Build history of the part. All positions in model axes, mm. A direction names the side the tool comes from. Round coordinates to 2 decimals unless told otherwise and drop trailing zeros. Write each loop counter-clockwise with the first axis right and the second up, starting at its lowest first coordinate (ties: lowest second). Pieces come first, ordered by that corner, then holes. Notation, with made-up numbers: (-9, 1.5) -> (38, 1.5) arc R12 ccw to (38, 23.5) -> close; hole circle Ø2 at (11.5, 88). An arc over 180 degrees is marked (long way). Answer in a Markdown table with one row per item.
```python
from build123d import *

# Parameters (mm, degrees)
F0_R     = 7.5
F1_DEPTH = 4
F2_R     = 5
F3_DEPTH = 100
F4_W     = 4
F4_H     = 4
F5_DEPTH = 20
F6_W     = 10.298821
F6_H     = 32.871584
F7_DEPTH = 25


with BuildPart() as f1:
    # F0 (on Top) → F1 (new body)
    with BuildSketch(Plane.XY):
        Circle(F0_R)
    extrude(amount=F1_DEPTH)

    # F2 (on Top) → F3 (join)
    with BuildSketch(Plane.XY):
        Circle(F2_R)
    extrude(amount=F3_DEPTH)

    # F4 (on face) → F5 (join)
    with BuildSketch(Plane.XY.offset(100)):
        Rectangle(F4_W, F4_H)
    extrude(amount=F5_DEPTH)

    # F6 (on Top) → F7 (cut)
    with BuildSketch(Plane.XY):
        with Locations((12.149411, 0.144365)):
            Rectangle(F6_W, F6_H)
    extrude(amount=F7_DEPTH, mode=Mode.SUBTRACT)


solid = f1.part
```
Q1. Saw through at D-D on x = -6. Write the cut outline in (y, z), plus the area to 3 significant figures.
A:
| item | result |
|---|---|
| outline | (-4.5, 0) -> (4.5, 0) -> (4.5, 4) -> (-4.5, 4) -> close |
| area | 36.0 mm² |
Q2. Which spindle directions (+Z, -Z, +X, -X, +Y, -Y) get a long thin tool onto all of the face, cutting with end or side? Do faces 1 (the flat face through (-5.2, 0.1, 4)), 2 (the flat face through (2, 0, 110)), 3 (the flat face through (-2, 0, 110)). Say none if no direction does.
A:
| item | result |
|---|---|
| face 1 | +Z |
| face 2 | +Z, +X, +Y, -Y |
| face 3 | +Z, -X, +Y, -Y |
Q3. Wall check: line 1 (Z direction, x = 1.75, y = -5); line 2 (Z direction, x = 3, y = -0.25); line 3 (Y direction, x = -4.5, z = 21.5). Give the ranges that are in metal, low to high. Write a range as [from, to].
A:
| item | result |
|---|---|
| line 1 | [0, 4] |
| line 2 | [0, 100] |
| line 3 | [-2.18, 2.18] |
Q4. Drop flat-ended pins along their axis: P1, Ø3, axis at y = -0.5, z = 110, coming from the +X side; P2, Ø6, axis at x = 3.5, z = 55.5, coming from the -Y side; P3, Ø2, axis at x = -0.5, z = 110.5, coming from the +Y side. Give the stop position or say it passes through.
A:
| item | result |
|---|---|
| P1 | x = 2 |
| P2 | y = -4.97 |
| P3 | y = 2 |
Q5. Saw through at C-C on z = 96. Write the cut outline in (x, y), plus the area to 3 significant figures.
A:
| item | result |
|---|---|
| outline | circle Ø10 at (0, 0) |
| area | 78.5 mm² |
Q6. Saw through at B-B on y = 0. Write the cut outline in (x, z), plus the area to 3 significant figures.
A:
| item | result |
|---|---|
| outline | (-7.5, 0) -> (7, 0) -> (7, 4) -> (5, 4) -> (5, 100) -> (2, 100) -> (2, 120) -> (-2, 120) -> (-2, 100) -> (-5, 100) -> (-5, 4) -> (-7.5, 4) -> close |
| area | 1,100 mm² |
Q7. Saw through at A-A on x = 0. Write the cut outline in (y, z).
A:
| item | result |
|---|---|
| outline | (-7.5, 0) -> (7.5, 0) -> (7.5, 4) -> (5, 4) -> (5, 100) -> (2, 100) -> (2, 120) -> (-2, 120) -> (-2, 100) -> (-5, 100) -> (-5, 4) -> (-7.5, 4) -> close |
Q8. Two-plate mould, pull along Z, no slides. Class faces 4 (the flat face through (0, 0, 0)), 5 (the cylindrical face through (-7.494, 0.291, 1.972)), 6 (the flat face through (0, 0, 120)): released by +Z, released by -Z, zero draft, split by the parting line, or undercut.
A:
| item | result |
|---|---|
| face 4 | released by -Z |
| face 5 | zero draft |
| face 6 | released by +Z |
